```python
from build123d import *

# Parameters (mm, degrees)
SKETCH1_R           = 5
SKETCH1_R_2         = 4.5
BOSS_EXTRUDE1_DEPTH = 350
SKETCH2_R           = 5
BOSS_EXTRUDE2_DEPTH = 30
SKETCH3_R           = 5
BOSS_EXTRUDE4_DEPTH = 30
SKETCH4_R           = 2.5
CUT_EXTRUDE1_DEPTH  = 15
SKETCH5_R           = 2.5
CUT_EXTRUDE2_DEPTH  = 15


with BuildPart() as part:
    # Sketch1 → Boss-Extrude1 (new body)
    with BuildSketch(Plane(origin=(0, 0, 0), x_dir=(1, 0, 0), z_dir=(0, 1, 0))):
        Circle(SKETCH1_R)
        Circle(SKETCH1_R_2, mode=Mode.SUBTRACT)
    extrude(amount=BOSS_EXTRUDE1_DEPTH)

    # Sketch2 → Boss-Extrude2 (add)
    with BuildSketch(Plane(origin=(0, 350, 0), x_dir=(1, 0, 0), z_dir=(0, 1, 0))):
        Circle(SKETCH2_R)
    extrude(amount=-BOSS_EXTRUDE2_DEPTH)

    # Sketch3 → Boss-Extrude4 (add)
    with BuildSketch(Plane(origin=(0, 0, 0), x_dir=(-1, 0, 0), z_dir=(0, -1, 0))):
        Circle(SKETCH3_R)
    extrude(amount=-BOSS_EXTRUDE4_DEPTH)

    # Sketch4 → Cut-Extrude1 (cut, symmetric)
    with BuildSketch(Plane(origin=(0, 0, 0), x_dir=(0, 0, -1), z_dir=(1, 0, 0))):
        with Locations((0, 10)):
            Circle(SKETCH4_R)
    extrude(amount=CUT_EXTRUDE1_DEPTH, both=True, mode=Mode.SUBTRACT)

    # Sketch5 → Cut-Extrude2 (cut, symmetric)
    with BuildSketch(Plane(origin=(0, 0, 0), x_dir=(0, 0, -1), z_dir=(1, 0, 0))):
        with Locations((0, 343.604340323)):
            Circle(SKETCH5_R)
    extrude(amount=CUT_EXTRUDE2_DEPTH, both=True, mode=Mode.SUBTRACT)


solid = part.part
```
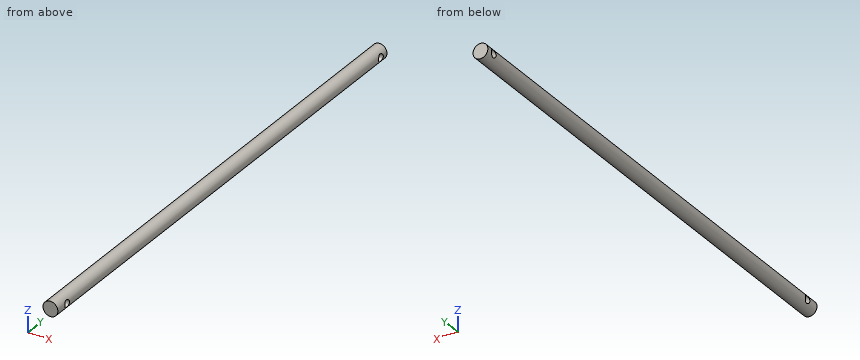
Model file for the job. Use its own axes, mm. Coordinates: 2 decimals unless noted, no trailing zeros. Order: outer loops, then holes, each group sorted by start corner. A loop starts at its lowest first (then second) coordinate and runs counter-clockwise, first axis right, second up. Notation, with made-up numbers: M 21,-27 L 66,-27 A28 ccw 66,-5 Z; hole C 62,76 d5. An arc over 180 degrees is marked long. Answer as CSV lines item,"result".
(1) Band-saw the part on B-B, the plane x = -1.25. List the corners of the cut face in (y, z), then the cut area to 3 significant figures.
Geometry says:
outline,"M 0,-4.84 L 350,-4.84 L 350,4.84 L 0,4.84 Z; hole C 10,0 d5; hole M 30,-4.32 L 320,-4.32 L 320,4.32 L 30,4.32 Z; hole C 343.6,0 d5"
area,"842 mm2"
(2) Wall check: line 1 along Y through (x, z) = (1.5, 0); line 2 along Y through (x, z) = (4.75, 0); line 3 along Z through (x, y) = (-0.25, 206). Give the ranges that are in metal, low to high.
Geometry says:
line 1,"y = 0 to 7.5, 12.5 to 30, 320 to 341.1, 346.1 to 350"
line 2,"y = 0 to 7.5, 12.5 to 341.1, 346.1 to 350"
line 3,"z = -4.99 to -4.49, 4.49 to 4.99"
(3) Band-saw the part on C-C, the plane y = 310.5. List the corners of the cut face in (x, z).
Geometry says:
outline,"C 0,0 d10; hole C 0,0 d9"
(4) Flat gauge pins, fed straight in: pin 1 (3 mm diameter, centred on x = 1, z = 1.5, fed in from -Y); pin 2 (3 mm diameter, centred on y = 69, z = 3.5, fed in from -X); pin 3 (5 mm diameter, centred on y = 157, z = -4, fed in from +X); pin 4 (1.5 mm diameter, centred on y = 219, z = 4, fed in from -X). Where does each tip first touch, or does it go through?
Geometry says:
pin 1,"stops at y = 0"
pin 2,"stops at x = -4.58"
pin 3,"stops at x = 4.77"
pin 4,"stops at x = -3.8"
(5) Band-saw the part on A-A, the plane z = 0. List the corners of the cut face in (x, y), then the cut area to 3 significant figures.
Geometry says:
outline,"M -5,0 L 5,0 L 5,7.5 L -5,7.5 Z; M -5,12.5 L 5,12.5 L 5,341.1 L -5,341.1 Z; M -5,346.1 L 5,346.1 L 5,350 L -5,350 Z; hole M -4.5,30 L 4.5,30 L 4.5,320 L -4.5,320 Z"
area,"790 mm2"
(6) Band-saw the part on D-D, the plane y = 25.5. List the corners of the cut face in (x, z).
Geometry says:
outline,"C 0,0 d10"
